Part print with two shaded views. Sizes in mm from the minimum x, y, z corner. A direction names the side the tool comes from. Coordinates: 2 decimals unless noted, no trailing zeros. Loops run counter-clockwise (first coordinate to the right, second up) from the corner with the lowest first, then second, coordinate; pieces in that order, holes last. Notation, with made-up numbers: (44, 81) -> (89, 81) arc R11 cw to (89, 95) -> close; hole circle Ø1 at (-7.75, 24). An arc over 180 degrees is marked (long way). One line per item, written item: value. Start each with the question number.
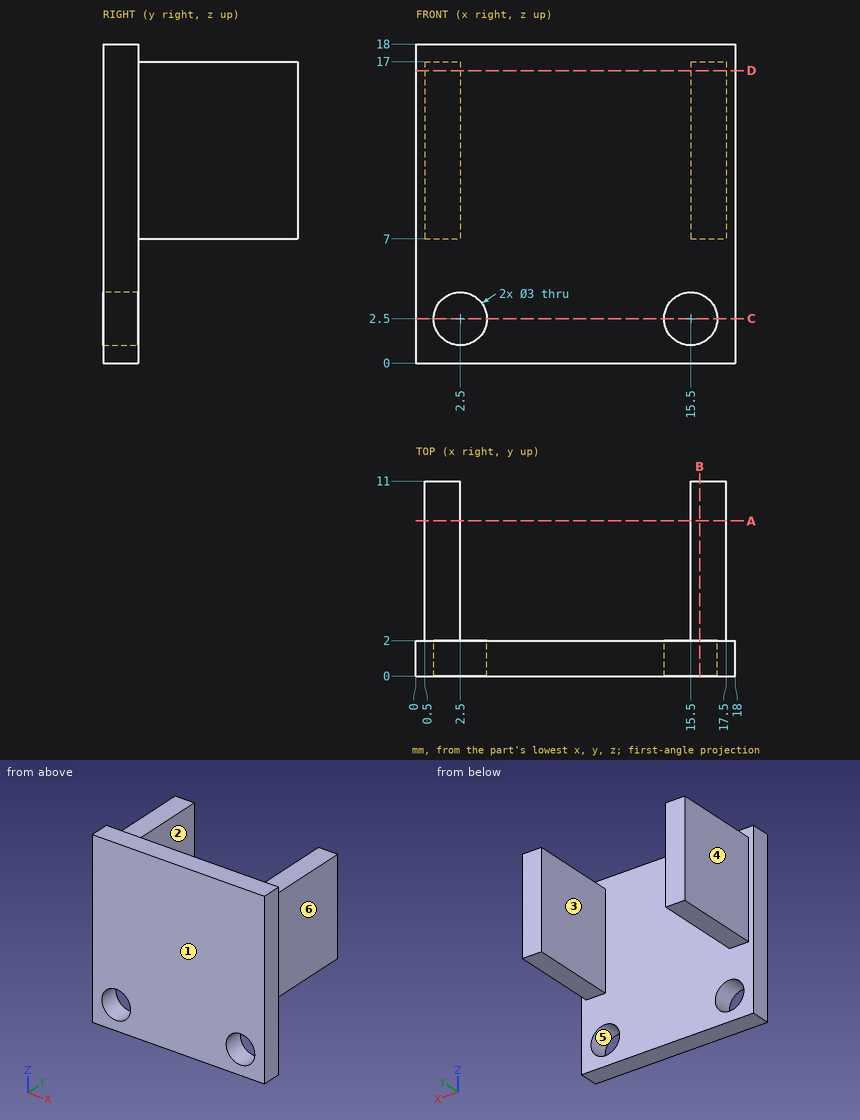
Item 1: Band-saw the part on A-A, the plane y = 8.75. List the corners of the cut face in (x, z), and give its area (3 significant figures).
Item 2: Tool access for the marked faces 5 and 6: list every direction of +Z, -Z, +X, -X, +Y, -Y with a clear straight run to the whole face (end or side of a thin tool).
Item 3: Two-plate mould, pull along X, no slides. Class the marked faces 1, 2, 3 and 4: +X half, -X half, draft (parallel to the pull), parting line (faces both ways), or undercut.
Item 4: Band-saw the part on D-D, the plane z = 16.5. List the corners of the cut face in (x, y), and give its area (3 significant figures).
Item 5: Drop flat-ended pins along their axis: pin 1 Ø1 at (x, y) = (16.5, 8) entering from -Z; pin 2 Ø1.6 at (x, y) = (16.5, 6) entering from +Z; pin 3 Ø2.5 at (y, z) = (8, 12.5) entering from +X. Give the stop position or say it passes through.
Item 6: Band-saw the part on C-C, the plane z = 2.5. List the corners of the cut face in (x, y), and give its area (3 significant figures).
Item 7: Band-saw the part on B-B, the plane x = 16. List the corners of the cut face in (y, z).
Item 8: Probe probe 1 along X at (y, z) = (0.55, 2.5); probe 2 along X at (y, z) = (4.25, 15.5); probe 3 along Y at (x, z) = (13, 4.75). List the from-to ranges inside material, lowest first.
Worked out:
1. outline: (0.5, 7) -> (2.5, 7) -> (2.5, 17) -> (0.5, 17) -> close; (15.5, 7) -> (17.5, 7) -> (17.5, 17) -> (15.5, 17) -> close
1. area: 40.0 mm²
2. face 5: +Y, -Y
2. face 6: +Z, -Z, +X, +Y
3. face 1: draft
3. face 2: undercut
3. face 3: undercut
3. face 4: -X half
4. outline: (0, 0) -> (18, 0) -> (18, 2) -> (17.5, 2) -> (17.5, 11) -> (15.5, 11) -> (15.5, 2) -> (2.5, 2) -> (2.5, 11) -> (0.5, 11) -> (0.5, 2) -> (0, 2) -> close
4. area: 72.0 mm²
5. pin 1: stops at z = 7
5. pin 2: stops at z = 17
5. pin 3: stops at x = 17.5
6. outline: (0, 0) -> (1, 0) -> (1, 2) -> (0, 2) -> close; (4, 0) -> (14, 0) -> (14, 2) -> (4, 2) -> close; (17, 0) -> (18, 0) -> (18, 2) -> (17, 2) -> close
6. area: 24.0 mm²
7. outline: (0, 0) -> (2, 0) -> (2, 1.09) -> (0, 1.09) -> close; (0, 3.91) -> (2, 3.91) -> (2, 7) -> (11, 7) -> (11, 17) -> (2, 17) -> (2, 18) -> (0, 18) -> close
8. probe 1: x = 0 to 1, 4 to 14, 17 to 18
8. probe 2: x = 0.5 to 2.5, 15.5 to 17.5
8. probe 3: y = 0 to 2
